The figure shows three views and two pictorial views of one solid part (mm, origin at its lowest corner). Answer the questions. A direction names the side the tool comes from. Give positions to 0.01 mm unless a question says otherwise; leave off trailing zeros. Write each loop counter-clockwise with the first axis right and the second up, starting at its lowest first coordinate (ties: lowest second). Pieces come first, ordered by that corner, then holes. Notation, with made-up numbers: (58.5, 35) -> (109.5, 35) arc R4 cw to (109.5, 41) -> close; hole circle Ø8 at (60.5, 71.5). An arc over 180 degrees is marked (long way). Write item = value, one per line. Start each with the question number.
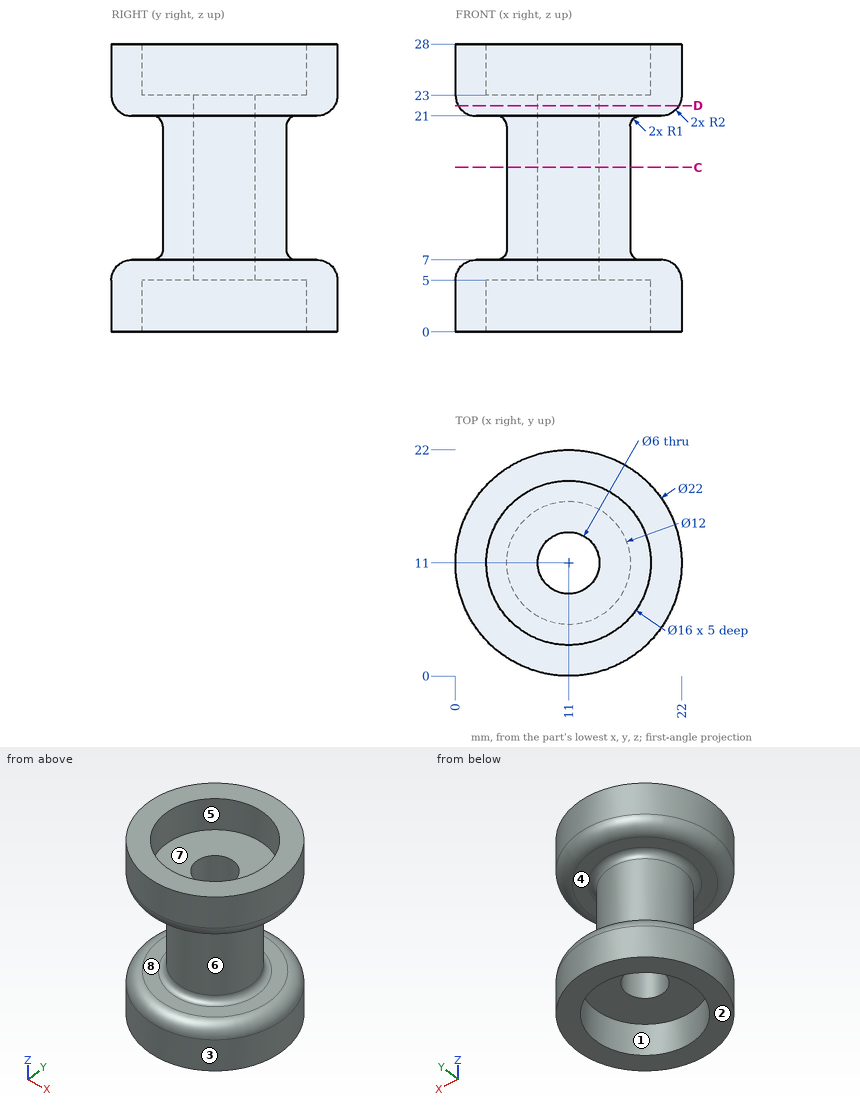
(1) Find the intervals of material crossed by line 1 along X through (y, z) = (11, 4); line 2 along Z through (x, y) = (17, 16.75); line 3 along Z through (x, y) = (12, 18), in increasing order.
(2) Each of these flat-tipped pins is pushed along its axis until it touches: pin 1 (10 mm diameter, centred on x = 15, z = 15, fed in from -Y); pin 2 (5 mm diameter, centred on x = 9.5, y = 11, fed in from -Z); pin 3 (1.5 mm diameter, centred on x = 14.5, z = 18, fed in from -Y); pin 4 (3.5 mm diameter, centred on x = 11, y = 11, fed in from +Z). Where does it stop, or does it pass through?
(3) A cutting plane is placed at D-D, the plane z = 22. Write down the section's boundary in (x, y).
(4) A cutting plane is placed at C-C, the plane z = 16. Write down the section's boundary in (x, y).
(5) Determine the mould class of the marked faces 6, 7 and 8 for opening direction X: pulls with the +X half, pulls with the -X half, needs draft (parallel to the pull), parting line crosses it, or undercut.
(6) For the marked faces 1, 2, 3, 4 and 5, determine the directions among +Z, -Z, +X, -X, +Y, -Y from which every point of the face is accessible in a straight line to the end or side of a thin tool.
Results list:
q1.line_1 = 0 to 3, 19 to 22
q1.line_2 = 0 to 7, 21 to 28
q1.line_3 = 5 to 7, 21 to 23
q2.pin_1 = 5
q2.pin_2 = 5
q2.pin_3 = 5.67
q2.pin_4 = through
q3.outline = circle Ø21.46 at (11, 11); hole circle Ø6 at (11, 11)
q4.outline = circle Ø12 at (11, 11); hole circle Ø6 at (11, 11)
q5.face_6 = parting line crosses it
q5.face_7 = undercut
q5.face_8 = needs draft
q6.face_1 = -Z
q6.face_2 = -Z, +X, -X, +Y, -Y
q6.face_3 = +Z, -Z
q6.face_4 = none
q6.face_5 = +Z
